Job drawing, mm, ordinate dimensions from the low corner. One solid piece. Give positions to 0.01 mm unless a question says otherwise; leave off trailing zeros. Write each loop counter-clockwise with the first axis right and the second up, starting at its lowest first coordinate (ties: lowest second). Pieces come first, ordered by that corner, then holes. Notation, with made-up numbers: M 62,8 L 66,8 A36 cw 66,46 Z; hole C 64.5,25.25 d11. An arc over 180 degrees is marked long. Answer as CSV lines item,"result". Start each with the question number.
Item 1: Band-saw the part on C-C, the plane x = 1763. List the corners of the cut face in (y, z), then the cut area to 3 significant figures.
Item 2: Band-saw the part on D-D, the plane z = 683.5. List the corners of the cut face in (x, y), then the cut area to 3 significant figures.
Item 3: Wall check: L1, parallel to Y at x = 1740, z = 677. Give the ranges that are in metal, low to high. Write a range as from..to.
Item 4: Band-saw the part on A-A, the plane z = 1000. List the corners of the cut face in (x, y).
Item 5: Pin check, flat tip, straight feed: pin 1 (8 mm diameter, centred on x = 925, z = 1114.5, fed in from +Y). Stop position of the tip, or through.
Item 6: Band-saw the part on B-B, the plane y = 277. List the corners of the cut face in (x, z), then the cut area to 3 significant figures.
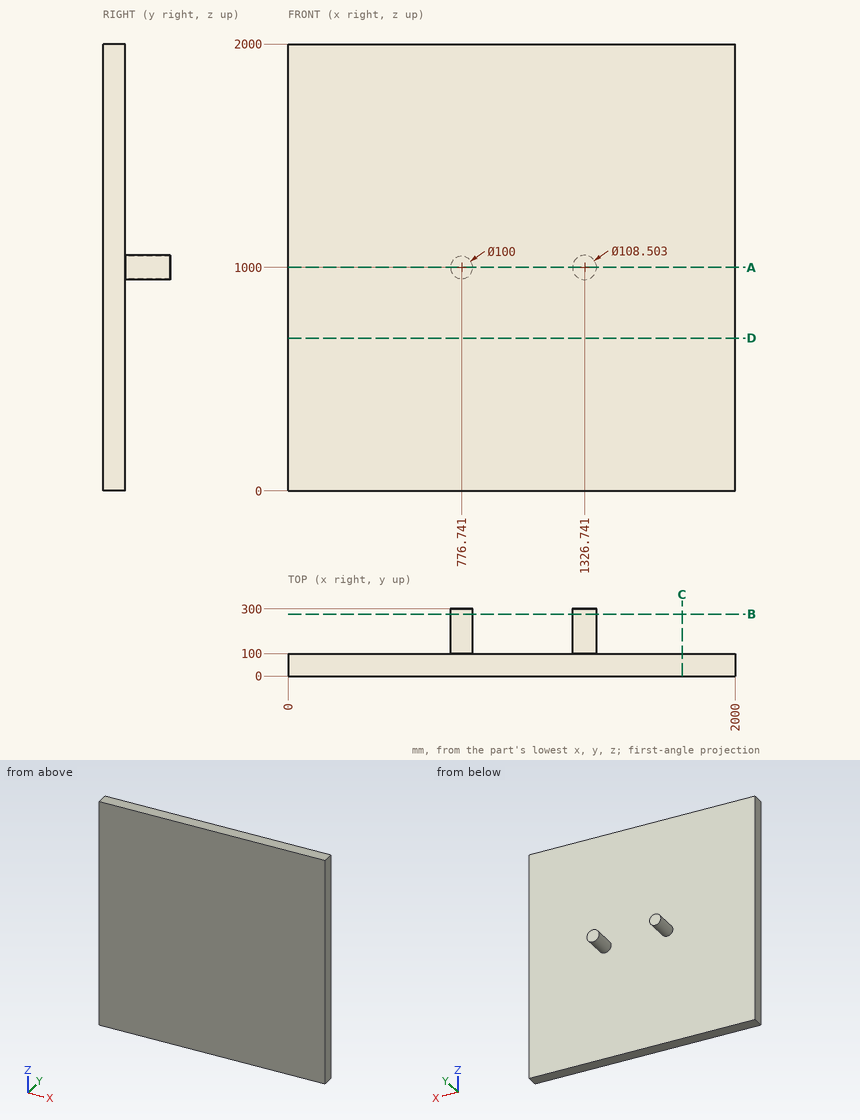
Output:
1,outline,"M 0,0 L 100,0 L 100,2000 L 0,2000 Z"
1,area,"200,000 mm²"
2,outline,"M 0,0 L 2000,0 L 2000,100 L 0,100 Z"
2,area,"200,000 mm²"
3,L1,"0..100"
4,outline,"M 0,0 L 2000,0 L 2000,100 L 1380.99,100 L 1380.99,300 L 1272.49,300 L 1272.49,100 L 826.74,100 L 826.74,300 L 726.74,300 L 726.74,100 L 0,100 Z"
5,pin 1,"y = 100"
6,outline,"C 776.74,1000 d100; C 1326.74,1000 d108.5"
6,area,"17,100 mm²"
